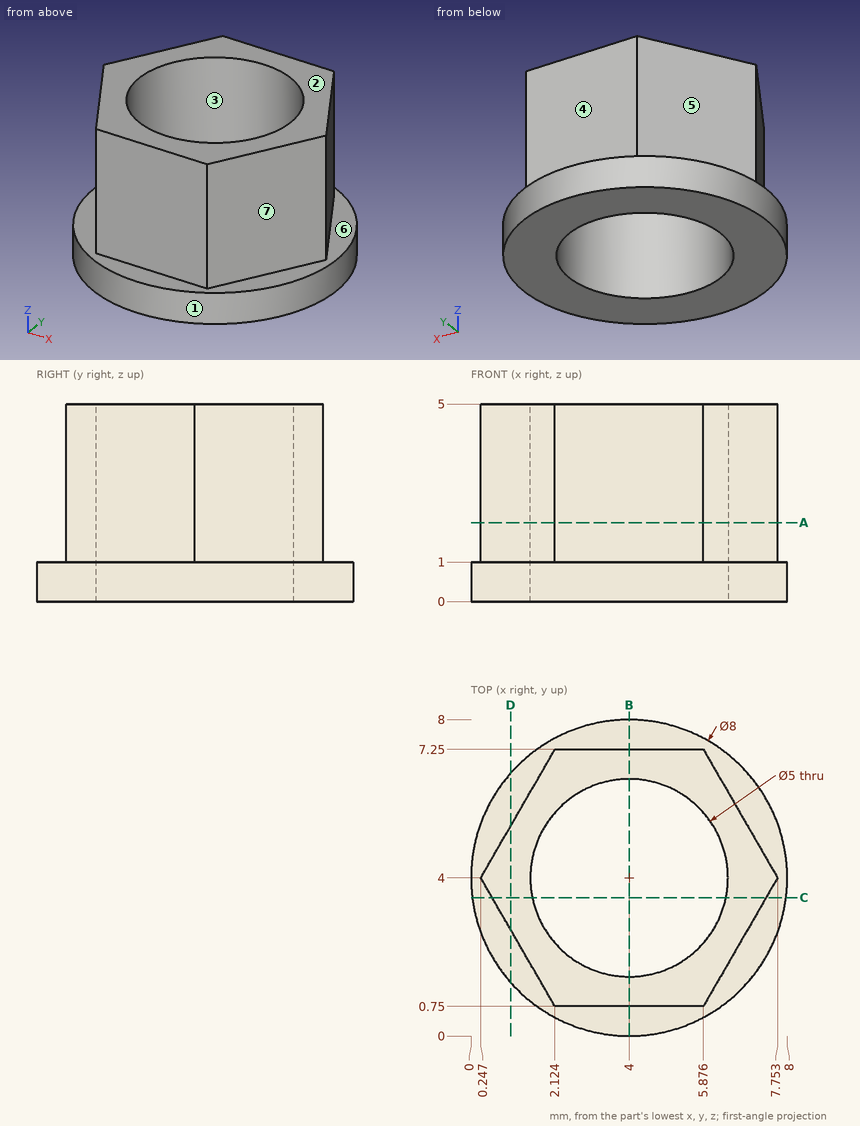
Job drawing, mm, ordinate dimensions from the low corner. One solid piece. A direction names the side the tool comes from. Round coordinates to 2 decimals unless told otherwise and drop trailing zeros. Loops run counter-clockwise (first coordinate to the right, second up) from the corner with the lowest first, then second, coordinate; pieces in that order, holes last.
Item 1: Cut at B-B, the plane x = 4. Give the cut face in (y, z).
Item 2: Mould opens along X. For the marked faces 1, 2 and 3 say: +X half, -X half, draft (parallel to the pull), parting line (faces both ways), or undercut.
Item 3: Cut at C-C, the plane y = 3.5. Give the cut face in (x, z).
Item 4: Drill centre lines: line 1 (Y direction, x = 4, z = 3.4); line 2 (Y direction, x = 2.5, z = 4.4); line 3 (Z direction, x = 3, y = 0.5). Where is each one in solid material? Low to high.
Item 5: Cut at A-A, the plane z = 2. Give the cut face in (x, y).
Item 6: Drop flat-ended pins along their axis: P1, Ø3, axis at y = 2, z = 2, coming from the -X side; P2, Ø1.9, axis at x = 3, z = 3.5, coming from the -Y side; P3, Ø1.1, axis at x = 3, z = 3, coming from the +Y side. Give the stop position or say it passes through.
Item 7: 3-axis set-ups, long thin cutter, end or side, ignore diameter. For the marked faces 4, 5, 6 and 7: which of +Z, -Z, +X, -X, +Y, -Y reach the whole face in a straight line?
Item 8: Cut at D-D, the plane x = 1. Give the cut face in (y, z) (1 decimal), then the cut area to 3 significant figures.
A:
1. outline: (0, 0) - (1.5, 0) - (1.5, 5) - (0.75, 5) - (0.75, 1) - (0, 1) - close; (6.5, 0) - (8, 0) - (8, 1) - (7.25, 1) - (7.25, 5) - (6.5, 5) - close
2. face 1: parting line
2. face 2: draft
2. face 3: undercut
3. outline: (0.03, 0) - (1.55, 0) - (1.55, 5) - (0.54, 5) - (0.54, 1) - (0.03, 1) - close; (6.45, 0) - (7.97, 0) - (7.97, 1) - (7.46, 1) - (7.46, 5) - (6.45, 5) - close
4. line 1: y = 0.75 to 1.5, 6.5 to 7.25
4. line 2: y = 0.75 to 2, 6 to 7.25
4. line 3: z = 0 to 1
5. outline: (0.25, 4) - (2.12, 0.75) - (5.88, 0.75) - (7.75, 4) - (5.88, 7.25) - (2.12, 7.25) - close; hole circle Ø5 at (4, 4)
6. P1: stops at x = 0.1
6. P2: stops at y = 0.75
6. P3: stops at y = 7.25
7. face 4: +Z, +X, -X, +Y
7. face 5: +Z, -X, +Y
7. face 6: +Z
7. face 7: +Z, +X, -Y
8. outline: (1.4, 0) - (6.6, 0) - (6.6, 1) - (5.3, 1) - (5.3, 5) - (2.7, 5) - (2.7, 1) - (1.4, 1) - close
8. area: 15.7 mm2
